Input: dimensioned drawing with shaded views. Units: mm. Origin: part minimum x, y, z. A direction names the side the tool comes from. Round coordinates to 2 decimals unless told otherwise and drop trailing zeros. Write each loop counter-clockwise with the first axis right and the second up, starting at its lowest first coordinate (ties: lowest second). Pieces come first, ordered by that corner, then holes. Notation, with made-up numbers: (32.5, 36.5) - (56.5, 36.5) arc R37 ccw to (56.5, 72.5) - close; hole circle Ø6 at (2, -21.5). An arc over 180 degrees is marked (long way). Write item = value, one per line. Start each with the question number.
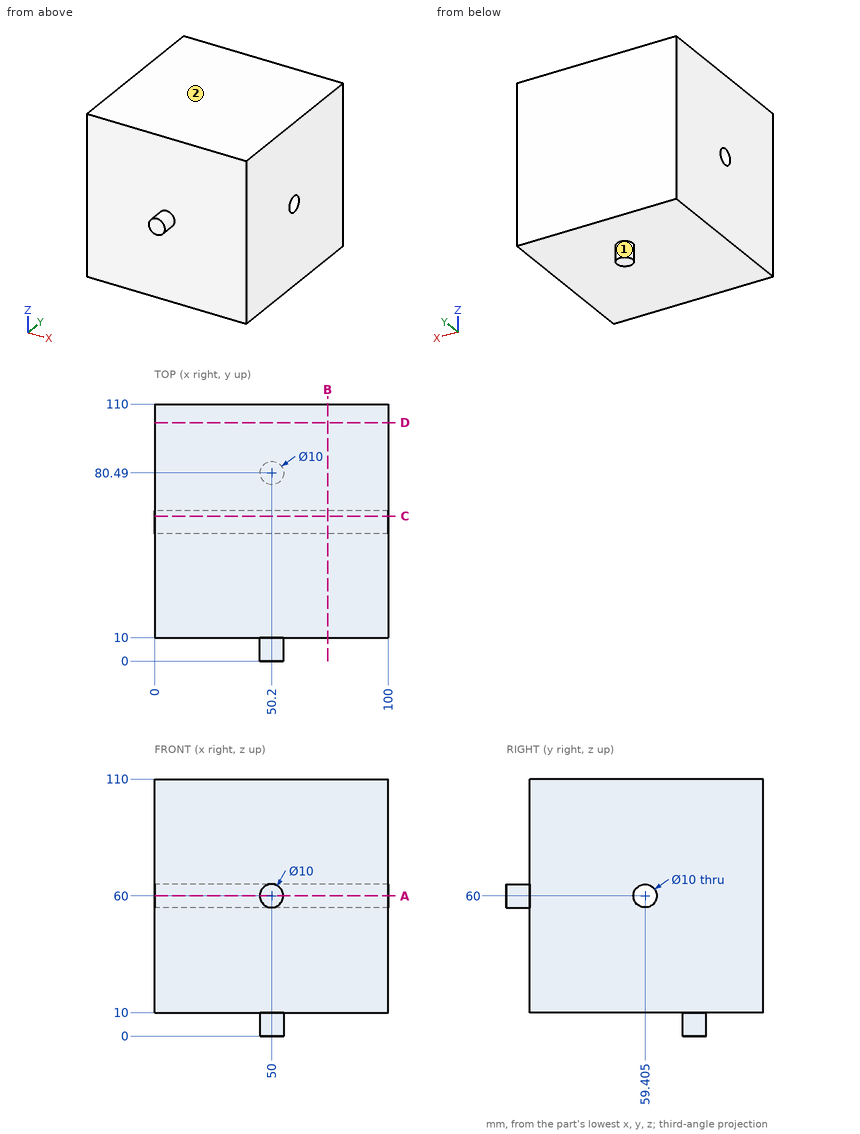
(1) Section D-D (y = 102). Return the cut outline in (x, z), plus the area to 3 significant figures.
(2) Contact query for flat-ended pins moving along their axis: P1, Ø1.5, axis at y = 53, z = 88.5, coming from the -X side; P2, Ø10, axis at x = 41, z = 97, coming from the -Y side; P3, Ø10, axis at x = 82.5, y = 25, coming from the -Z side. Output: stop coordinate, or through.
(3) Section C-C (y = 62). Return the cut outline in (x, z).
(4) Ray query, L1, parallel to Z at x = 50, y = 89.5; L2, parallel to Z at x = 53, y = 61. Return the intervals inside material, ascending. Write a range as from..to.
(5) Section B-B (x = 74). Return the cut outline in (y, z) (1 decimal).
(6) Reachability of the marked faces 1 and 2 from +Z, -Z, +X, -X, +Y, -Y: full face, straight path, thin tool, end or side. Return the list, or none.
(7) Section A-A (z = 60). Return the cut outline in (x, y) (1 decimal).
Solution:
q1.outline = (0, 10) - (100, 10) - (100, 110) - (0, 110) - close
q1.area = 10,000 mm^2
q2.P1 = 0
q2.P2 = 10
q2.P3 = 10
q3.outline = (0, 10) - (100, 10) - (100, 55.73) - (0, 55.73) - close; (0, 64.27) - (100, 64.27) - (100, 110) - (0, 110) - close
q4.L1 = 10..110
q4.L2 = 10..55.26, 64.74..110
q5.outline = (10, 10) - (110, 10) - (110, 110) - (10, 110) - close; hole circle Ø10 at (59.4, 60)
q6.face_1 = -Z
q6.face_2 = +Z, +X, -X, +Y, -Y
q7.outline = (0, 10) - (45, 10) - (45, 0) - (55, 0) - (55, 10) - (100, 10) - (100, 54.4) - (0, 54.4) - close; (0, 64.4) - (100, 64.4) - (100, 110) - (0, 110) - close
